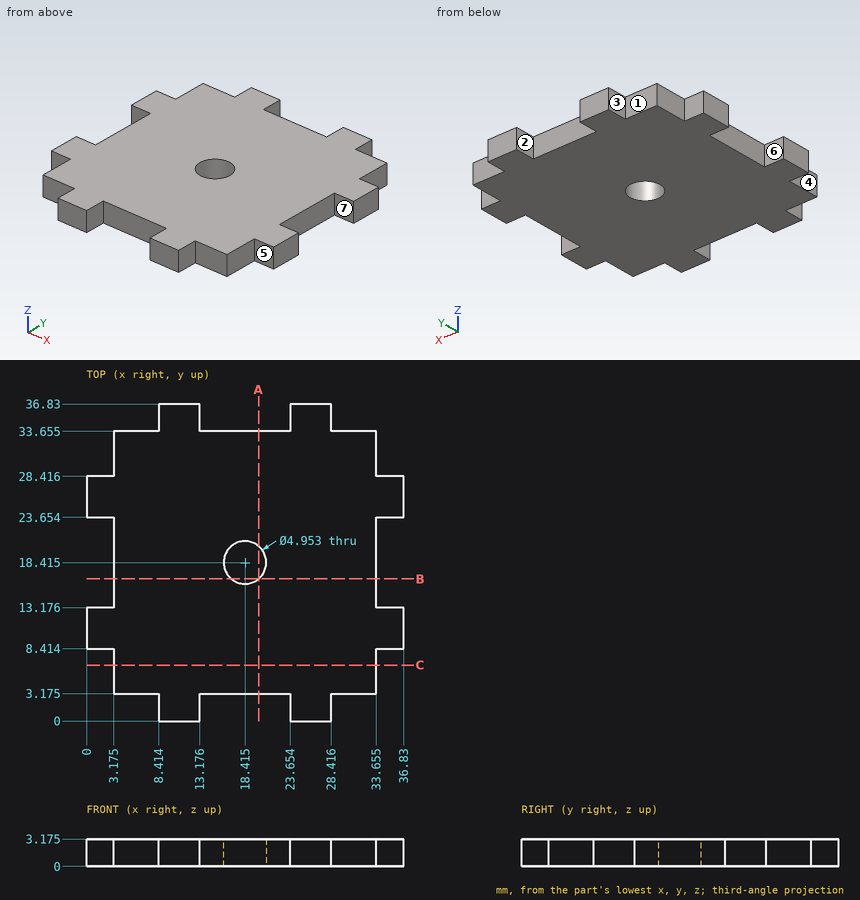
Job drawing, mm, ordinate dimensions from the low corner. One solid piece. A direction names the side the tool comes from. Round coordinates to 2 decimals unless told otherwise and drop trailing zeros. Loops run counter-clockwise (first coordinate to the right, second up) from the corner with the lowest first, then second, coordinate; pieces in that order, holes last. Notation, with made-up numbers: (-10, -39.5) -> (19, -39.5) arc R22 ccw to (19, -31.5) -> close; hole circle Ø8 at (45.5, 10). An arc over 180 degrees is marked (long way). One line per item, written item: value. Start each with the question number.
Q1. Two-plate mould, pull along X, no slides. Class the marked faces 1, 2 and 3: released by +X, released by -X, zero draft, split by the parting line, or undercut.
Q2. Probe line 1 along Y through (x, z) = (31, 0.35) (1 decimal); line 2 along Y through (x, z) = (35.5, 0.4). List the from-to ranges inside material, lowest first.
Q3. Cut at A-A on x = 20. List the corners of the cut face in (y, z) (1 decimal).
Q4. Drop flat-ended pins along their axis: pin 1 Ø1 at (x, z) = (18, 1) entering from +Y (3 decimals); pin 2 Ø1 at (y, z) = (31, 1.5) entering from -X (3 decimals); pin 3 Ø1 at (y, z) = (22.5, 1) entering from +X (3 decimals); pin 4 Ø5.5 at (x, y) = (18.415, 18.415) entering from -Z. Give the stop position or say it passes through.
Q5. Cut at C-C on y = 6.5. List the corners of the cut face in (x, z) (1 decimal).
Q6. Cut at B-B on y = 16.5. List the corners of the cut face in (x, z) (1 decimal).
Q7. 3-axis set-ups, long thin cutter, end or side, ignore diameter. For the marked faces 4, 5, 6 and 7: which of +Z, -Z, +X, -X, +Y, -Y reach the whole face in a straight line?
Computed:
1. face 1: zero draft
1. face 2: undercut
1. face 3: released by -X
2. line 1: 3.2 to 33.7
2. line 2: 8.41 to 13.18, 23.65 to 28.42
3. outline: (3.2, 0) -> (16.5, 0) -> (16.5, 3.2) -> (3.2, 3.2) -> close; (20.3, 0) -> (33.7, 0) -> (33.7, 3.2) -> (20.3, 3.2) -> close
4. pin 1: y = 33.655
4. pin 2: x = 3.175
4. pin 3: x = 33.655
4. pin 4: z = 0
5. outline: (3.2, 0) -> (33.7, 0) -> (33.7, 3.2) -> (3.2, 3.2) -> close
6. outline: (3.2, 0) -> (16.8, 0) -> (16.8, 3.2) -> (3.2, 3.2) -> close; (20, 0) -> (33.7, 0) -> (33.7, 3.2) -> (20, 3.2) -> close
7. face 4: +Z, -Z, -X, -Y
7. face 5: +Z, -Z, +X, -Y
7. face 6: +Z, -Z, -X
7. face 7: +Z, -Z, +X
